```python
from build123d import *

# Parameters (mm, degrees)
SKETCH1_R           = 22.5
BOSS_EXTRUDE1_DEPTH = 20
CUT_EXTRUDE2_DEPTH  = 20


with BuildPart() as part:
    # Sketch1 → Boss-Extrude1 (new body)
    with BuildSketch(Plane(origin=(0, 0, 0), x_dir=(1, 0, 0), z_dir=(0, 1, 0))):
        Circle(SKETCH1_R)
    extrude(amount=BOSS_EXTRUDE1_DEPTH)

    # Sketch2 → Cut-Extrude2 (cut)
    with BuildSketch(Plane(origin=(0, 20, 0), x_dir=(1, 0, 0), z_dir=(0, 1, 0))):
        with BuildLine():
            Line((5, -2.5), (5, 2.5))
            Line((5, 2.5), (9.682458366, 2.5))
            ThreePointArc((9.682458366, 2.5), (-10, 0), (9.682458366, -2.5))
            Line((9.682458366, -2.5), (5, -2.5))
        make_face()
        with BuildLine():
            Line((9.682458366, 2.5), (5, 2.5))
            Line((5, 2.5), (5, -2.5))
            Line((5, -2.5), (9.682458366, -2.5))
            ThreePointArc((9.682458366, -2.5), (9.920296963, -1.260042925), (10, 0))
            ThreePointArc((10, 0), (9.920296963, 1.260042925), (9.682458366, 2.5))
        make_face()
        with BuildLine():
            Line((15, 2.5), (9.682458366, 2.5))
            ThreePointArc((9.682458366, 2.5), (9.920296963, 1.260042925), (10, 0))
            ThreePointArc((10, 0), (9.920296963, -1.260042925), (9.682458366, -2.5))
            Line((9.682458366, -2.5), (15, -2.5))
            Line((15, -2.5), (15, 2.5))
        make_face()
    extrude(amount=-CUT_EXTRUDE2_DEPTH, mode=Mode.SUBTRACT)


solid = part.part
```
Could you check a few things on this model? Use its own coordinates, in mm. A direction names the side the tool comes from. Coordinates: 2 decimals unless noted, no trailing zeros. Order: outer loops, then holes, each group sorted by start corner. A loop starts at its lowest first (then second) coordinate and runs counter-clockwise, first axis right, second up. Notation, with made-up numbers: M 47,29 L 85,29 A15 ccw 85,34 Z; hole C 10,0 d3. An arc over 180 degrees is marked long. Use a Markdown table: item, result. Add a question column.
Q1. I'm going to push flat-ended pins straight in: pin 1 (3 mm diameter, centred on x = -3.5, y = 5, fed in from -Z); pin 2 (1.6 mm diameter, centred on x = 13, y = 14, fed in from -Z); pin 3 (1 mm diameter, centred on y = 17.5, z = -10.5, fed in from +X); pin 4 (23 mm diameter, centred on x = 0, z = 0, fed in from +Y). Where does each tip first touch, or does it pass through?
Q2. I want a section at B-B on x = 0. List the corners of the cut face in (y, z) for me.
Q3. If I drill on L1, parallel to Z at x = 0, y = 7.25; L2, parallel to X at y = 6, z = 0; L3, parallel to Z at x = 2, y = 1.5, over which ranges is the centre line in solid material (lowest first)?
Q4. I want a section at A-A on z = 0. List the corners of the cut face in (x, y) for me, then the cut area to 3 significant figures.
Q5. I want a section at C-C on y = 17. List the corners of the cut face in (x, z) for me.
Q6. We'd pull the mould along X, two halves only. Please class faces 3 (the cylindrical face through (10.382, 9.86, 19.961)), 4 (the flat face through (15, 10, 0)), 5 (the flat face through (-10.3, 0, -0.3)): pulls with the +X half, pulls with the -X half, needs draft (parallel to the pull), parting line crosses it, or undercut.
Q7. Which directions (+Z, -Z, +X, -X, +Y, -Y) give clear straight access to the entire face, cutting with the end or side of a thin tool? Please do faces 1 (the flat face through (-10.3, 20, -0.3)), 2 (the flat face through (12, 10, -2.5)).
Q8. I want a section at D-D on x = 18. List the corners of the cut face in (y, z) for me.
Checked values:
| question | item | result |
|---|---|---|
| 1 | pin 1 | z = -22.41 |
| 1 | pin 2 | z = -18.91 |
| 1 | pin 3 | x = 20.16 |
| 1 | pin 4 | y = 20 |
| 2 | outline | M 0,-22.5 L 20,-22.5 L 20,-10 L 0,-10 Z; M 0,10 L 20,10 L 20,22.5 L 0,22.5 Z |
| 3 | L1 | -22.5 to -10, 10 to 22.5 |
| 3 | L2 | -22.5 to -10, 15 to 22.5 |
| 3 | L3 | -22.41 to -9.8, 9.8 to 22.41 |
| 4 | outline | M -22.5,0 L -10,0 L -10,20 L -22.5,20 Z; M 15,0 L 22.5,0 L 22.5,20 L 15,20 Z |
| 4 | area | 400 mm² |
| 5 | outline | C 0,0 d45; hole M 9.68,-2.5 L 15,-2.5 L 15,2.5 L 9.68,2.5 A10 ccw long Z |
| 6 | face 3 | parting line crosses it |
| 6 | face 4 | undercut |
| 6 | face 5 | needs draft |
| 7 | face 1 | +Z, -Z, +X, -X, +Y |
| 7 | face 2 | +Y, -Y |
| 8 | outline | M 0,-13.5 L 20,-13.5 L 20,13.5 L 0,13.5 Z |
